from build123d import *

# Parameters (mm, degrees)
SKETCH1_R           = 1
BOSS_EXTRUDE1_DEPTH = 8
SKETCH2_W           = 63
SKETCH2_H           = 15
BOSS_EXTRUDE2_DEPTH = 2
SKETCH3_R           = 1.7
CUT_EXTRUDE1_DEPTH  = 2
SKETCH4_W           = 41
SKETCH4_H           = 45
CUT_EXTRUDE2_DEPTH  = 5
SKETCH5_W           = 65
SKETCH5_H           = 21.051864014
CUT_EXTRUDE3_DEPTH  = 5


with BuildPart() as part:
    # Sketch1 → Boss-Extrude1 (new body)
    with BuildSketch(Plane(origin=(0, 0, 0), x_dir=(1, 0, 0), z_dir=(0, 1, 0))):
        with BuildLine():
            Line((-28.5, 22.5), (28.5, 22.5))
            ThreePointArc((28.5, 22.5), (31.328427125, 21.328427125), (32.5, 18.5))
            Line((32.5, 18.5), (32.5, -18.5))
            ThreePointArc((32.5, -18.5), (31.328427125, -21.328427125), (28.5, -22.5))
            Line((28.5, -22.5), (-28.5, -22.5))
            ThreePointArc((-28.5, -22.5), (-31.328427125, -21.328427125), (-32.5, -18.5))
            Line((-32.5, -18.5), (-32.5, 18.5))
            ThreePointArc((-32.5, 18.5), (-31.328427125, 21.328427125), (-28.5, 22.5))
        make_face()
        with Locations(Location((-25, 14.25, 0), (0, 0, 270))):
            Circle(SKETCH1_R, mode=Mode.SUBTRACT)
        with Locations(Location((25, 14.25, 0), (0, 0, 270))):
            Circle(SKETCH1_R, mode=Mode.SUBTRACT)
        with Locations(Location((25, -14.25, 0), (0, 0, 270))):
            Circle(SKETCH1_R, mode=Mode.SUBTRACT)
        with Locations(Location((-25, -14.25, 0), (0, 0, 270))):
            Circle(SKETCH1_R, mode=Mode.SUBTRACT)
        with BuildLine():
            Line((-30.5, 10.5), (-30.5, -10.5))
            Line((-30.5, -10.5), (-24.5, -10.5))
            ThreePointArc((-24.5, -10.5), (-21.671572875, -11.671572875), (-20.5, -14.5))
            Line((-20.5, -14.5), (-20.5, -20.5))
            Line((-20.5, -20.5), (20.5, -20.5))
            Line((20.5, -20.5), (20.5, -14.5))
            ThreePointArc((20.5, -14.5), (21.671572875, -11.671572875), (24.5, -10.5))
            Line((24.5, -10.5), (30.5, -10.5))
            Line((30.5, -10.5), (30.5, 10.5))
            Line((30.5, 10.5), (24.5, 10.5))
            ThreePointArc((24.5, 10.5), (21.671572875, 11.671572875), (20.5, 14.5))
            Line((20.5, 14.5), (20.5, 20.5))
            Line((20.5, 20.5), (-20.5, 20.5))
            Line((-20.5, 20.5), (-20.5, 14.5))
            ThreePointArc((-20.5, 14.5), (-21.671572875, 11.671572875), (-24.5, 10.5))
            Line((-24.5, 10.5), (-30.5, 10.5))
        make_face(mode=Mode.SUBTRACT)
    extrude(amount=BOSS_EXTRUDE1_DEPTH)

    # Sketch2 → Boss-Extrude2 (add)
    with BuildSketch(Plane(origin=(0, 0, 0), x_dir=(1, 0, 0), z_dir=(0, 1, 0))):
        Rectangle(SKETCH2_W, SKETCH2_H)
    extrude(amount=BOSS_EXTRUDE2_DEPTH)

    # Sketch3 → Cut-Extrude1 (cut)
    with BuildSketch(Plane(origin=(0, 2, 0), x_dir=(1, 0, 0), z_dir=(0, 1, 0))):
        with Locations(Location((-20, 0, 0), (0, 0, 270))):
            Circle(SKETCH3_R)
        with Locations(Location((20, 0, 0), (0, 0, 270))):
            Circle(SKETCH3_R)
    extrude(amount=-CUT_EXTRUDE1_DEPTH, mode=Mode.SUBTRACT)

    # Sketch4 → Cut-Extrude2 (cut)
    with BuildSketch(Plane(origin=(0, 8, 0), x_dir=(1, 0, 0), z_dir=(0, 1, 0))):
        Rectangle(SKETCH4_W, SKETCH4_H)
    extrude(amount=-CUT_EXTRUDE2_DEPTH, mode=Mode.SUBTRACT)

    # Sketch5 → Cut-Extrude3 (cut)
    with BuildSketch(Plane(origin=(0, 8, 0), x_dir=(1, 0, 0), z_dir=(0, 1, 0))):
        with Locations((0, -0.025932007)):
            Rectangle(SKETCH5_W, SKETCH5_H)
    extrude(amount=-CUT_EXTRUDE3_DEPTH, mode=Mode.SUBTRACT)


solid = part.part
Input: part model. Units: mm. Frame: model coordinates. A direction names the side the tool comes from. Coordinates: 2 decimals unless noted, no trailing zeros. Loops run counter-clockwise (first coordinate to the right, second up) from the corner with the lowest first, then second, coordinate; pieces in that order, holes last. Notation, with made-up numbers: (-27, -32.75) -> (-20, -32.75) arc R33 cw to (-20, 3.25) -> close; hole circle Ø10 at (-4.75, -14). An arc over 180 degrees is marked (long way). Write item = value, one per line. Start each with the question number.
Item 1: Reachability of faces 1 (the face through (-31.359, 3.944, -21.297)), 2 (the face through (30.5, 2.5, 0.1)), 3 (the face through (-28, 6, 10.552)), 4 (the face through (-28, 1, 10.5)) from +Z, -Z, +X, -X, +Y, -Y: full face, straight path, thin tool, end or side. Return the list, or none.
Item 2: Cut plane A-A, the plane x = -6. Return loops of the section in (y, z), plus the area to 3 significant figures.
Item 3: Cut plane D-D, the plane z = -6.5. Return loops of the section in (x, y), plus the area to 3 significant figures.
Item 4: Material intervals for line 1 (X direction, y = 4.75, z = -14.25); line 2 (Z direction, x = 12.5, y = 0.5); line 3 (X direction, y = 1.15, z = 0), sorted ascending.
Item 5: First-contact query: P1, Ø4.5, axis at x = 30, z = 3.5, coming from the +Y side; P2, Ø4, axis at y = 2.5, z = 20.5, coming from the -X side; P3, Ø1.2, axis at x = 25, z = 14.25, coming from the +Y side; P4, Ø4.5, axis at x = -28, z = -1, coming from the +Y side. Flat tips, straight axial feed; report the tip coordinate or a pass-through.
Item 6: Cut plane C-C, the plane z = -1. Return loops of the section in (x, y), plus the area to 3 significant figures.
Item 7: Cut plane B-B, the plane y = 4. Return loops of the section in (x, z), plus the area to 3 significant figures.
Item 8: Mould query, pull axis Z, two halves, no side actions, for faces 5 (the face through (-26, 8, -17)), 6 (the face through (0, 2, -22.5)), 7 (the face through (0, 2, 22.5)), 8 (the face through (0, 1, -7.5)). Classes: pulls with the +Z half, pulls with the -Z half, needs draft (parallel to the pull), parting line crosses it, or undercut.
Ans:
q1.face_1 = -Z, -X, +Y, -Y
q1.face_2 = +Y
q1.face_3 = +X, -X, +Y
q1.face_4 = +Y, -Y
q2.outline = (0, -22.5) -> (3, -22.5) -> (3, -20.5) -> (0, -20.5) -> close; (0, -7.5) -> (2, -7.5) -> (2, 7.5) -> (0, 7.5) -> close; (0, 20.5) -> (3, 20.5) -> (3, 22.5) -> (0, 22.5) -> close
q2.area = 42.0 mm²
q3.outline = (-32.5, 0) -> (32.5, 0) -> (32.5, 3) -> (30.5, 3) -> (30.5, 2) -> (-30.5, 2) -> (-30.5, 3) -> (-32.5, 3) -> close
q3.area = 134 mm²
q4.line_1 = -32.5 to -26, -24 to -20.51, 20.51 to 24, 26 to 32.5
q4.line_2 = -22.5 to -20.5, -7.5 to 7.5, 20.5 to 22.5
q4.line_3 = -32.5 to -21.7, -18.3 to 18.3, 21.7 to 32.5
q5.P1 = 3
q5.P2 = -32.5
q5.P3 = through
q5.P4 = 2
q6.outline = (-32.5, 0) -> (-21.37, 0) -> (-21.37, 2) -> (-30.5, 2) -> (-30.5, 3) -> (-32.5, 3) -> close; (-18.63, 0) -> (18.63, 0) -> (18.63, 2) -> (-18.63, 2) -> close; (21.37, 0) -> (32.5, 0) -> (32.5, 3) -> (30.5, 3) -> (30.5, 2) -> (21.37, 2) -> close
q6.area = 123 mm²
q7.outline = (-32.5, -18.5) arc R4 ccw to (-28.5, -22.5) -> (-20.5, -22.5) -> (-20.5, -14.5) arc R4 ccw to (-24.5, -10.5) -> (-32.5, -10.5) -> close; (-32.5, 10.55) -> (-23.86, 10.55) arc R4 ccw to (-20.5, 14.5) -> (-20.5, 22.5) -> (-28.5, 22.5) arc R4 ccw to (-32.5, 18.5) -> close; (20.5, -22.5) -> (28.5, -22.5) arc R4 ccw to (32.5, -18.5) -> (32.5, -10.5) -> (24.5, -10.5) arc R4 ccw to (20.5, -14.5) -> close; (20.5, 14.5) arc R4 ccw to (23.86, 10.55) -> (32.5, 10.55) -> (32.5, 18.5) arc R4 ccw to (28.5, 22.5) -> (20.5, 22.5) -> close; hole circle Ø2 at (-25, -14.25); hole circle Ø2 at (-25, 14.25); hole circle Ø2 at (25, -14.25); hole circle Ø2 at (25, 14.25)
q7.area = 535 mm²
q8.face_5 = needs draft
q8.face_6 = pulls with the -Z half
q8.face_7 = pulls with the +Z half
q8.face_8 = undercut
